Part model, mm, in its own coordinate system. Face numbers are marked on the shaded views. A direction names the side the tool comes from. Round coordinates to 2 decimals unless told otherwise and drop trailing zeros. Loops run counter-clockwise (first coordinate to the right, second up) from the corner with the lowest first, then second, coordinate; pieces in that order, holes last. Notation, with made-up numbers: M 47,88.25 L 70,88.25 A18 cw 70,100.25 Z; hole C -27.75,-32 d4. An arc over 180 degrees is marked long. Put each result on its own line as item: value. Start each with the question number.
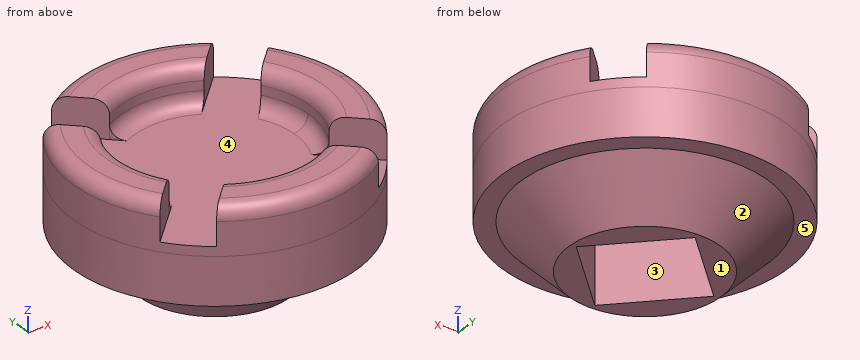
```python
from build123d import *

# Parameters (mm, degrees)
SKETCH_1_R          = 1.599999994
EXTRUDE_1_DEPTH     = 2
SKETCH_2_R          = 3
EXTRUDE_2_DEPTH     = 1
SKETCH_3_R          = 3
SKETCH_3_R_2        = 1.599999994
EXTRUDE_3_DEPTH     = 1
CUT_EXTRUDE_1_DEPTH = 0.8
SKETCH_5_R          = 2
CUT_EXTRUDE_2_DEPTH = 0.8
FILLET_1_R          = 0.3
FILLET_2_R          = 0.3
CHAMFER_2_SIZE      = 1
EXTRUDE_4_DEPTH     = 0.5


# Some blends are built 0.0001 mm under size
with BuildPart() as part:
    # 草图1 → 凸台-拉伸1 (new body)
    with BuildSketch(Plane.XY):
        Circle(SKETCH_1_R)
        Polygon((1.484924235, 0), (0, 1.484924235), (-1.484924235, 0), (0, -1.484924235), align=None, mode=Mode.SUBTRACT)
    extrude(amount=-EXTRUDE_1_DEPTH)

    # 草图2 → 凸台-拉伸2 (add)
    with BuildSketch(Plane.XY):
        Circle(SKETCH_2_R)
    extrude(amount=EXTRUDE_2_DEPTH)

    # 草图3 → 凸台-拉伸3 (add)
    with BuildSketch(Plane(origin=(0, 0, 0), x_dir=(-1, 0, 0), z_dir=(0, 0, -1))):
        Circle(SKETCH_3_R)
        with Locations(Location((0, 0, 0), (0, 0, 180))):
            Circle(SKETCH_3_R_2, mode=Mode.SUBTRACT)
    extrude(amount=EXTRUDE_3_DEPTH)

    # 草图4 → 切除-拉伸1 (cut)
    with BuildSketch(Plane.XY.offset(1)):
        Polygon((2.840154811, -2.105592708), (2.13698266, -2.816612347), (0.001071679, -0.704275308), (-2.12840084, -2.823102879), (-2.833733613, -2.114226528), (-0.709971025, -0.001080346), (-2.840154811, 2.105592708), (-2.13698266, 2.816612347), (-0.001071679, 0.704275308), (2.12840084, 2.823102879), (2.833733613, 2.114226528), (0.709971025, 0.001080346), align=None)
    extrude(amount=-CUT_EXTRUDE_1_DEPTH, mode=Mode.SUBTRACT)

    # 草图5 → 切除-拉伸2 (cut)
    with BuildSketch(Plane.XY.offset(1)):
        Circle(SKETCH_5_R)
    extrude(amount=-CUT_EXTRUDE_2_DEPTH, mode=Mode.SUBTRACT)

    # 圆角1
    fillet_1_edges = [part.edges().sort_by_distance(p)[0] for p in [
        (1.930129409, 0.524023343, 1),
        (0.003043349, -1.999997685, 1),
        (-1.999997685, -0.003043349, 1),
        (-0.003043349, 1.999997685, 1),
        (-0.004565023, 2.999996527, 1),
        (-2.999996527, -0.004565023, 1),
        (0.004565023, -2.999996527, 1),
        (2.859077887, 0.908665855, 1),
    ]]
    fillet(fillet_1_edges, radius=FILLET_1_R)

    # 圆角2
    # the kernel refuses this fillet: 0.3 mm, written as the material it adds along each edge
    with BuildSketch(Plane(origin=(0, 0, 0.2), x_dir=(0.7896841124236736, 0.613513653137104, 0), z_dir=(0.613513653137104, -0.7896841124236736, 0))) as fillet_2_piece_1_section:
        with BuildLine():
            CenterArc((2 - FILLET_2_R, FILLET_2_R), FILLET_2_R, 270, 90)
            Line((2 - FILLET_2_R, 0), (2, 0))
            Line((2, 0), (2, FILLET_2_R))
        make_face()
    fillet_2_piece_1 = revolve(axis=Axis((0, 0, 0.2), (0, 0, 1)), revolution_arc=104.486373309, mode=Mode.PRIVATE)
    fillet_2_piece_1 = split(fillet_2_piece_1, bisect_by=Plane(origin=(0.603196481, 1.305522812, 0.285319886), z_dir=(-0.7053327724211024, 0.7088763503945956, 0)), keep=Keep.TOP, mode=Mode.PRIVATE)
    fillet_2_piece_1 = split(fillet_2_piece_1, bisect_by=Plane(origin=(-0.607166844, 1.303681031, 0.285319886), z_dir=(0.7031721506430704, 0.711019638659861, 0)), keep=Keep.TOP, mode=Mode.PRIVATE)
    add(fillet_2_piece_1)
    with BuildSketch(Plane(origin=(0, 0, 0.2), x_dir=(1, 0, 0), z_dir=(0, -1, 0))) as fillet_2_piece_2_section:
        with BuildLine():
            CenterArc((2 - FILLET_2_R, FILLET_2_R), FILLET_2_R, 270, 90)
            Line((2 - FILLET_2_R, 0), (2, 0))
            Line((2, 0), (2, FILLET_2_R))
        make_face()
    fillet_2_piece_2 = revolve(axis=Axis((0, 0, 0.2), (0, 0, 1)), revolution_arc=51.865822775, mode=Mode.PRIVATE)
    fillet_2_piece_2 = split(fillet_2_piece_2, bisect_by=Plane(origin=(1.528365858, 0.815384132, 0.269855635), z_dir=(0.7053327724211024, -0.7088763503945955, 0)), keep=Keep.TOP, mode=Mode.PRIVATE)
    add(fillet_2_piece_2)
    with BuildSketch(Plane(origin=(0, 0, 0.2), x_dir=(-0.7896841124236732, -0.6135136531371046, 0), z_dir=(-0.6135136531371046, 0.7896841124236732, 0))) as fillet_2_piece_3_section:
        with BuildLine():
            CenterArc((2 - FILLET_2_R, FILLET_2_R), FILLET_2_R, 270, 90)
            Line((2 - FILLET_2_R, 0), (2, 0))
            Line((2, 0), (2, FILLET_2_R))
        make_face()
    fillet_2_piece_3 = revolve(axis=Axis((0, 0, 0.2), (0, 0, 1)), revolution_arc=104.486373309, mode=Mode.PRIVATE)
    fillet_2_piece_3 = split(fillet_2_piece_3, bisect_by=Plane(origin=(0.607166844, -1.303681031, 0.285319886), z_dir=(-0.7031721506430706, -0.7110196386598608, 0)), keep=Keep.TOP, mode=Mode.PRIVATE)
    fillet_2_piece_3 = split(fillet_2_piece_3, bisect_by=Plane(origin=(-0.603196481, -1.305522812, 0.285319886), z_dir=(0.7053327724211026, -0.7088763503945954, 0)), keep=Keep.TOP, mode=Mode.PRIVATE)
    add(fillet_2_piece_3)
    with BuildSketch(Plane(origin=(0, 0, 0.2), x_dir=(-0.6198560202042671, 0.784715562619047, 0), z_dir=(0.784715562619047, 0.6198560202042671, 0))) as fillet_2_piece_4_section:
        with BuildLine():
            CenterArc((2 - FILLET_2_R, FILLET_2_R), FILLET_2_R, 270, 90)
            Line((2 - FILLET_2_R, 0), (2, 0))
            Line((2, 0), (2, FILLET_2_R))
        make_face()
    fillet_2_piece_4 = revolve(axis=Axis((0, 0, 0.2), (0, 0, 1)), revolution_arc=103.563128964, mode=Mode.PRIVATE)
    fillet_2_piece_4 = split(fillet_2_piece_4, bisect_by=Plane(origin=(-1.316253088, -0.604331686, 0.285332918), z_dir=(-0.7053327724211024, 0.7088763503945957, 0)), keep=Keep.TOP, mode=Mode.PRIVATE)
    fillet_2_piece_4 = split(fillet_2_piece_4, bisect_by=Plane(origin=(-1.318086183, 0.600323075, 0.285332918), z_dir=(-0.7031721506430707, -0.7110196386598606, 0)), keep=Keep.TOP, mode=Mode.PRIVATE)
    add(fillet_2_piece_4)
    with BuildSketch(Plane(origin=(0, 0, 0.2), x_dir=(0.6198962648649622, -0.7846837712139004, 0), z_dir=(-0.7846837712139004, -0.6198962648649622, 0))) as fillet_2_piece_5_section:
        with BuildLine():
            CenterArc((2 - FILLET_2_R, FILLET_2_R), FILLET_2_R, 270, 90)
            Line((2 - FILLET_2_R, 0), (2, 0))
            Line((2, 0), (2, FILLET_2_R))
        make_face()
    fillet_2_piece_5 = revolve(axis=Axis((0, 0, 0.2), (0, 0, 1)), revolution_arc=51.69144042, mode=Mode.PRIVATE)
    fillet_2_piece_5 = split(fillet_2_piece_5, bisect_by=Plane(origin=(1.532032043, -0.811907626, 0.269859578), z_dir=(0.7031721506430706, 0.7110196386598608, 0)), keep=Keep.TOP, mode=Mode.PRIVATE)
    add(fillet_2_piece_5)

    # 倒角2
    chamfer_2_edges = [part.edges().sort_by_distance(p)[0] for p in [
        (-1.599999994, 0, -1),
    ]]
    chamfer(chamfer_2_edges, length=CHAMFER_2_SIZE - 0.0001)  # a hair under: the kernel refuses the full size

    # 草图6 → 凸台-拉伸4 (add)
    with BuildSketch(Plane(origin=(0, 0, 0), x_dir=(-1, 0, 0), z_dir=(0, 0, -1))):
        Polygon((0, 1.484924235), (1.484924235, 0), (0, -1.484924235), (-1.484924235, 0), align=None)
    extrude(amount=EXTRUDE_4_DEPTH)


solid = part.part
```
1. Cut at A-A, the plane z = 0.3. Give the cut face in (x, y).
2. Which spindle directions (+Z, -Z, +X, -X, +Y, -Y) get a long thin tool onto all of the face, cutting with end or side? Do the marked faces 4 and 5. Say none if no direction does.
3. Mould opens along Y. For the marked faces 1, 2 and 3 say: released by +Y, released by -Y, zero draft, split by the parting line, or undercut.
4. Wall check: L1, parallel to Y at x = -1.5, z = -0.1; L2, parallel to Y at x = 1.25, z = -0.9; L3, parallel to X at y = -1.25, z = -1.2. Give the ranges that are in metal, low to high.
5. Drop a flat-ended pin along its axis: pin 1 (1.5 mm diameter, centred on y = -1.5, z = -1, fed in from +X). Give the stop position or say it passes through.
Results list:
1. outline: M -2.45,-1.73 L -1.67,-0.96 A1.92 cw -1.67,0.95 L -2.45,1.72 A3 ccw Z; M -1.75,2.44 L -0.97,1.66 A1.92 cw 0.96,1.66 L 1.74,2.44 A3 ccw Z; M -1.74,-2.44 A3 ccw 1.75,-2.44 L 0.97,-1.66 A1.92 cw -0.96,-1.66 Z; M 1.67,-0.95 L 2.45,-1.72 A3 ccw 2.45,1.73 L 1.67,0.96 A1.92 cw Z
2. face 4: +Z
2. face 5: -Z
3. face 1: zero draft
3. face 2: split by the parting line
3. face 3: undercut
4. L1: y = -2.6 to 2.6
4. L2: y = -2.73 to -0.23, 0.23 to 2.73
4. L3: x = -2.05 to -0.23, 0.23 to 2.05
5. pin 1: stops at x = 2.9
